Print and shaded views of the part. All mm, measured from the part's lowest x, y and z. A direction names the side the tool comes from. Round coordinates to 2 decimals unless told otherwise and drop trailing zeros. Loops run counter-clockwise (first coordinate to the right, second up) from the corner with the lowest first, then second, coordinate; pieces in that order, holes last. Notation, with made-up numbers: (44.25, 70) -> (81.25, 70) arc R21 ccw to (81.25, 106) -> close; hole circle Ø3 at (65, -8.5). An arc over 180 degrees is marked (long way). Answer as CSV lines item,"result".
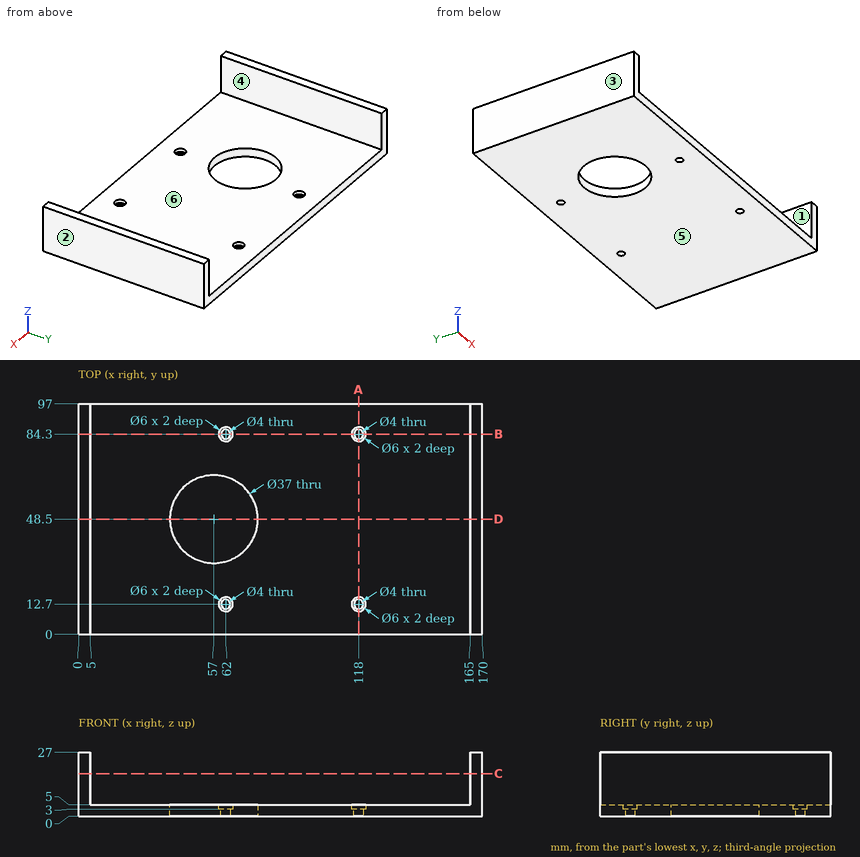
Q1. Which spindle directions (+Z, -Z, +X, -X, +Y, -Y) get a long thin tool onto all of the face, cutting with end or side? Do the marked faces 1 and 2. Say none if no direction does.
Geometry results:
face 1,"+Z, +Y, -Y"
face 2,"+Z, -Z, +X, +Y, -Y"
Q2. Saw through at C-C, the plane z = 18. Write the cut outline in (x, y), then the cut area to 3 significant figures.
Geometry results:
outline,"(0, 0) -> (5, 0) -> (5, 97) -> (0, 97) -> close; (165, 0) -> (170, 0) -> (170, 97) -> (165, 97) -> close"
area,"970 mm2"
Q3. Two-plate mould, pull along X, no slides. Class the marked faces 3, 4, 5 and 6: pulls with the +X half, pulls with the -X half, needs draft (parallel to the pull), parting line crosses it, or undercut.
Geometry results:
face 3,"pulls with the -X half"
face 4,"undercut"
face 5,"needs draft"
face 6,"undercut"
Q4. Saw through at B-B, the plane y = 84.3. Write the cut outline in (x, z), then the cut area to 3 significant figures.
Geometry results:
outline,"(0, 0) -> (60, 0) -> (60, 3) -> (59, 3) -> (59, 5) -> (5, 5) -> (5, 27) -> (0, 27) -> close; (64, 0) -> (116, 0) -> (116, 3) -> (115, 3) -> (115, 5) -> (65, 5) -> (65, 3) -> (64, 3) -> close; (120, 0) -> (170, 0) -> (170, 27) -> (165, 27) -> (165, 5) -> (121, 5) -> (121, 3) -> (120, 3) -> close"
area,"1,020 mm2"
Q5. Saw through at A-A, the plane x = 118. Write the cut outline in (y, z).
Geometry results:
outline,"(0, 0) -> (10.7, 0) -> (10.7, 3) -> (9.7, 3) -> (9.7, 5) -> (0, 5) -> close; (14.7, 0) -> (82.3, 0) -> (82.3, 3) -> (81.3, 3) -> (81.3, 5) -> (15.7, 5) -> (15.7, 3) -> (14.7, 3) -> close; (86.3, 0) -> (97, 0) -> (97, 5) -> (87.3, 5) -> (87.3, 3) -> (86.3, 3) -> close"
Q6. Drop flat-ended pins along their axis: P1, Ø1.8, axis at x = 61, y = 83.5, coming from the +Z side; P2, Ø7, axis at x = 118, y = 84.3, coming from the +Z side. Give the stop position or say it passes through.
Geometry results:
P1,"z = 3"
P2,"z = 5"
Q7. Drill centre lines: line 1 along Y through (x, z) = (118, 3.8); line 2 along X through (y, z) = (19, 25); line 3 along Y through (x, z) = (118, 2.25). Where is each one in solid material? Low to high.
Geometry results:
line 1,"0 to 9.7, 15.7 to 81.3, 87.3 to 97"
line 2,"0 to 5, 165 to 170"
line 3,"0 to 10.7, 14.7 to 82.3, 86.3 to 97"
Q8. Saw through at D-D, the plane y = 48.5. Write the cut outline in (x, z).
Geometry results:
outline,"(0, 0) -> (38.5, 0) -> (38.5, 5) -> (5, 5) -> (5, 27) -> (0, 27) -> close; (75.5, 0) -> (170, 0) -> (170, 27) -> (165, 27) -> (165, 5) -> (75.5, 5) -> close"
